```python
from build123d import *

# Parameters (mm, degrees)
SKETCH2_W           = 184.3
SKETCH2_H           = 19.3
BOSS_EXTRUDE1_DEPTH = 15
SHELL1_T            = -2
FILLET1_R           = 3
FILLET2_R           = 1.5
CHAMFER1_SIZE       = 1


with BuildPart() as part:
    # Sketch2 → Boss-Extrude1 (new body)
    with BuildSketch(Plane(origin=(0, 0, 0), x_dir=(1, 0, 0), z_dir=(0, 1, 0))):
        Rectangle(SKETCH2_W, SKETCH2_H)
    extrude(amount=BOSS_EXTRUDE1_DEPTH)

    # Shell1
    shell1_openings = [part.faces().sort_by_distance(p)[0] for p in [
        (0, 15, 0),
    ]]
    offset(amount=SHELL1_T, openings=shell1_openings, kind=Kind.INTERSECTION)

    # Fillet1
    fillet1_edges = [part.edges().sort_by_distance(p)[0] for p in [
        (0, 0, 9.65),
        (-92.15, 0, 0),
        (0, 0, -9.65),
        (92.15, 0, 0),
        (92.15, 7.5, 9.65),
        (-92.15, 7.5, 9.65),
        (-92.15, 7.5, -9.65),
        (92.15, 7.5, -9.65),
    ]]
    fillet(fillet1_edges, radius=FILLET1_R)

    # Fillet2
    fillet2_edges = [part.edges().sort_by_distance(p)[0] for p in [
        (90.15, 8.5, 7.65),
        (90.15, 8.5, -7.65),
        (-90.15, 8.5, -7.65),
        (-90.15, 8.5, 7.65),
    ]]
    fillet(fillet2_edges, radius=FILLET2_R)

    # Chamfer1
    chamfer1_edges = [part.edges().sort_by_distance(p)[0] for p in [
        (0, 15, 7.65),
        (90.15, 15, 0),
        (0, 15, -7.65),
        (-90.15, 15, 0),
        (89.710660172, 15, 7.210660172),
        (89.710660172, 15, -7.210660172),
        (-89.710660172, 15, 7.210660172),
        (-89.710660172, 15, -7.210660172),
    ]]
    chamfer(chamfer1_edges, length=CHAMFER1_SIZE)


solid = part.part
```
Here's how the part is built. I have some questions about the finished solid (model axes, mm). A direction names the side the tool comes from. Give positions to 0.01 mm unless a question says otherwise; leave off trailing zeros. Order: outer loops, then holes, each group sorted by start corner. A loop starts at its lowest first (then second) coordinate and runs counter-clockwise, first axis right, second up. Notation, with made-up numbers: M 89,-25 L 120,-25 A31 ccw 120,-1 Z; hole C 67,29 d2. An arc over 180 degrees is marked long. Use a Markdown table: item, result. Add a question column.
1. For pin 1 Ø3 at (x, z) = (16, -1.5) entering from +Y, with a flat end and sliding along its axis, tell me the tip position at first contact or that it passes through.
2. I need wall thicknesses on probe 1 along Z at (x, y) = (-8, 7.75); probe 2 along X at (y, z) = (7.25, 6). Which ranges of each line are inside material? Lowest first, please. Write a range as from..to.
3. On a 3-axis mill with a long thin cutter (end or side, diameter ignored), from which of +Z, -Z, +X, -X, +Y, -Y can I reach the whole of each face in a straight line? I mean faces 5 (the flat face through (-1, 2, 0)), 6 (the cylindrical face through (91.25, 9.08, 8.79)). Say none if no direction works.
4. Suppose I cut it at B-B (x = -74). List the corners of the cut face in (y, z) for me, and give its area (3 significant figures).
5. Suppose I cut it at A-A (y = 11.25). List the corners of the cut face in (x, z) for me, and give its area (3 significant figures).
6. Suppose I cut it at C-C (z = 2.5). List the corners of the cut face in (x, y) for me, and give its area (3 significant figures).
7. If we mould it in two halves opening along Z, with no side actions, what happens to faces 1 (the flat face through (0, 15, -9)), 2 (the flat face through (-1, 8, 7.65)), 3 (the cylindrical face through (1.25, 0.9, 8.79)), 4 (the flat face through (-1, 8, -7.65))? For each: +Z half, -Z half, draft (parallel to the pull), parting line (faces both ways), or undercut.
Results list:
| question | item | result |
|---|---|---|
| 1 | pin 1 | stops at y = 2 |
| 2 | probe 1 | z = -9.65..-7.65, 7.65..9.65 |
| 2 | probe 2 | x = -92.15..-90.15, 90.15..92.15 |
| 3 | face 5 | +Y |
| 3 | face 6 | +Z, +X, +Y, -Y |
| 4 | outline | M 0,-6.65 A3 ccw 3,-9.65 L 15,-9.65 L 15,-8.65 L 14,-7.65 L 2,-7.65 L 2,7.65 L 14,7.65 L 15,8.65 L 15,9.65 L 3,9.65 A3 ccw 0,6.65 Z |
| 4 | area | 85.7 mm² |
| 5 | outline | M -92.15,-6.65 A3 ccw -89.15,-9.65 L 89.15,-9.65 A3 ccw 92.15,-6.65 L 92.15,6.65 A3 ccw 89.15,9.65 L -89.15,9.65 A3 ccw -92.15,6.65 Z; hole M -90.15,-6.15 A1.5 ccw -88.65,-7.65 L 88.65,-7.65 A1.5 ccw 90.15,-6.15 L 90.15,6.15 A1.5 ccw 88.65,7.65 L -88.65,7.65 A1.5 ccw -90.15,6.15 Z |
| 5 | area | 793 mm² |
| 6 | outline | M -92.15,3 A3 ccw -89.15,0 L 89.15,0 A3 ccw 92.15,3 L 92.15,15 L 91.15,15 L 90.15,14 L 90.15,2 L -90.15,2 L -90.15,14 L -91.15,15 L -92.15,15 Z |
| 6 | area | 416 mm² |
| 7 | face 1 | draft |
| 7 | face 2 | undercut |
| 7 | face 3 | +Z half |
| 7 | face 4 | undercut |
